Check sheet for the modelled part. Datum: model origin and axes. Units: mm. Coordinates: 2 decimals unless noted, no trailing zeros. Write each loop counter-clockwise with the first axis right and the second up, starting at its lowest first coordinate (ties: lowest second). Pieces come first, ordered by that corner, then holes. Notation, with made-up numbers: M -3.75,11 L 5.25,11 A13 cw 5.25,19 Z; hole C 86.25,-0.75 d1. An arc over 180 degrees is marked long. Answer as CSV lines item,"result". Start each with the question number.
Q1. Sectioned sample at B-B, the plane z = 58.5. Record the cut outline in (x, y), then the cut area to 3 significant figures.
Q2. Sectioned sample at A-A, the plane x = -0.5. Record the cut outline in (y, z), then the cut area to 3 significant figures.
Q3. Sectioned sample at D-D, the plane z = -27.5. Record the cut outline in (x, y), then the cut area to 3 significant figures.
Q4. Thickness scan on line 1 along Z through (x, y) = (-1.5, 0.8); line 2 along X through (y, z) = (1.75, -75) (3 decimals); line 3 along X through (y, z) = (1.85, 75). Record the ranges inside material, lowest first. Write a range as from..to.
Q5. Depth check by flat-ended pin: pin 1 Ø1.6 at (y, z) = (1, -76.5) entering from -X; pin 2 Ø1.6 at (y, z) = (2, -31) entering from +X. Enter the tip coordinate at first touch or a pass-through.
Q6. Sectioned sample at C-C, the plane x = 14.5. Record the cut outline in (y, z), then the cut area to 4 significant figures.
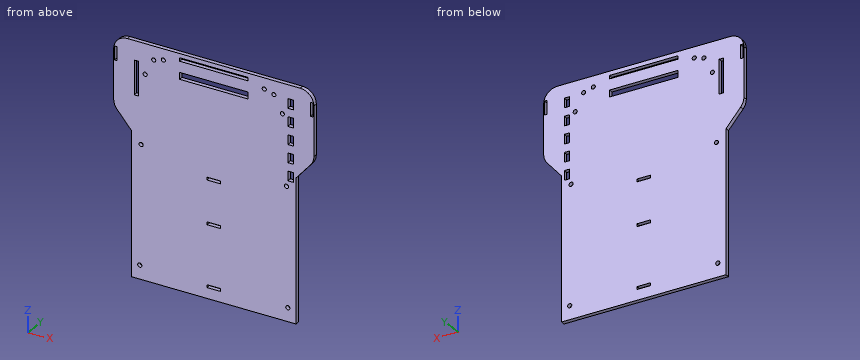
from build123d import *

# Parameters (mm, degrees)
BOSS_EXTRUDE1_DEPTH = 3
SKETCH2_R           = 1.525
CUT_EXTRUDE1_DEPTH  = 113.084789334
SKETCH3_W           = 10
SKETCH3_H           = 2.05
CUT_EXTRUDE2_DEPTH  = 113.084789334
SKETCH4_R           = 1.5
CUT_EXTRUDE3_DEPTH  = 3
SKETCH5_R           = 1.5
SKETCH5_W           = 50
SKETCH5_H           = 5
CUT_EXTRUDE4_DEPTH  = 3
SKETCH6_W           = 4
SKETCH6_H           = 7
CUT_EXTRUDE5_DEPTH  = 10
SKETCH7_W           = 50
SKETCH7_H           = 2.5
SKETCH7_W_2         = 3.05
SKETCH7_H_2         = 25
CUT_EXTRUDE6_DEPTH  = 10
FILLET3_R           = 10
SKETCH8_W           = 2
SKETCH8_H           = 10
CUT_EXTRUDE7_DEPTH  = 10


with BuildPart() as part:
    # Sketch1 → Boss-Extrude1 (new body)
    with BuildSketch(Plane(origin=(0, 0, 0), x_dir=(1, 0, 0), z_dir=(0, 1, 0))):
        Polygon((-73, -35), (-60, -19.801315846), (-60, 85), (60, 85), (60, -19.801315846), (73, -35), (73, -85), (60, -85), (-60, -85), (-73, -85), align=None)
    extrude(amount=BOSS_EXTRUDE1_DEPTH)

    # Sketch2 → Cut-Extrude1 (cut, through all)
    with BuildSketch(Plane(origin=(0, 3, 0), x_dir=(1, 0, 0), z_dir=(0, 1, 0))):
        with Locations(Location((-53, -11.81, 0), (0, 0, 270))):
            Circle(SKETCH2_R)
        with Locations(Location((-54, 75, 0), (0, 0, 270))):
            Circle(SKETCH2_R)
        with Locations(Location((53, -11.81, 0), (0, 0, 90))):
            Circle(SKETCH2_R)
        with Locations(Location((54, 75, 0), (0, 0, 90))):
            Circle(SKETCH2_R)
    extrude(amount=-CUT_EXTRUDE1_DEPTH, mode=Mode.SUBTRACT)

    # Sketch3 → Cut-Extrude2 (cut, through all)
    with BuildSketch(Plane(origin=(0, 3, 0), x_dir=(1, 0, 0), z_dir=(0, 1, 0))):
        with Locations((0, 31.115)):
            Rectangle(SKETCH3_W, SKETCH3_H)
        with Locations((0, -0.985)):
            Rectangle(SKETCH3_W, SKETCH3_H)
        with Locations((0, 76.215)):
            Rectangle(SKETCH3_W, SKETCH3_H)
    extrude(amount=-CUT_EXTRUDE2_DEPTH, mode=Mode.SUBTRACT)

    # Sketch4 → Cut-Extrude3 (cut)
    with BuildSketch(Plane(origin=(0, 3, 0), x_dir=(1, 0, 0), z_dir=(0, 1, 0))):
        with Locations(Location((-50, -63, 0), (0, 0, 270))):
            Circle(SKETCH4_R)
        with Locations(Location((-43.815341562, -75, 0), (0, 0, 270))):
            Circle(SKETCH4_R)
        with Locations(Location((43.815341562, -75, 0), (0, 0, 90))):
            Circle(SKETCH4_R)
        with Locations(Location((50, -63, 0), (0, 0, 90))):
            Circle(SKETCH4_R)
    extrude(amount=-CUT_EXTRUDE3_DEPTH, mode=Mode.SUBTRACT)

    # Sketch5 → Cut-Extrude4 (cut)
    with BuildSketch(Plane(origin=(0, 3, 0), x_dir=(1, 0, 0), z_dir=(0, 1, 0))):
        with Locations(Location((-36.8, -77, 0), (0, 0, 270))):
            Circle(SKETCH5_R)
        with Locations(Location((36.8, -77, 0), (0, 0, 90))):
            Circle(SKETCH5_R)
        with Locations((0, -69)):
            Rectangle(SKETCH5_W, SKETCH5_H)
    extrude(amount=-CUT_EXTRUDE4_DEPTH, mode=Mode.SUBTRACT)

    # Sketch6 → Cut-Extrude5 (cut)
    with BuildSketch(Plane(origin=(0, 3, 0), x_dir=(1, 0, 0), z_dir=(0, 1, 0))):
        with Locations((56, -32.549614417)):
            Rectangle(SKETCH6_W, SKETCH6_H)
        with Locations((56, -19.549614417)):
            Rectangle(SKETCH6_W, SKETCH6_H)
        with Locations((56, -45.549614417)):
            Rectangle(SKETCH6_W, SKETCH6_H)
        with Locations((56, -58.549614417)):
            Rectangle(SKETCH6_W, SKETCH6_H)
        with Locations((56, -71.549614417)):
            Rectangle(SKETCH6_W, SKETCH6_H)
    extrude(amount=-CUT_EXTRUDE5_DEPTH, mode=Mode.SUBTRACT)

    # Sketch7 → Cut-Extrude6 (cut)
    with BuildSketch(Plane(origin=(0, 3, 0), x_dir=(1, 0, 0), z_dir=(0, 1, 0))):
        with Locations((0, -80.75)):
            Rectangle(SKETCH7_W, SKETCH7_H)
        with Locations((-56.475, -58.5)):
            Rectangle(SKETCH7_W_2, SKETCH7_H_2)
    extrude(amount=-CUT_EXTRUDE6_DEPTH, mode=Mode.SUBTRACT)

    # Fillet3
    fillet3_edges = [part.edges().sort_by_distance(p)[0] for p in [
        (73, 1.5, 35),
        (73, 1.5, 85),
        (-73, 1.5, 85),
        (-73, 1.5, 35),
    ]]
    fillet(fillet3_edges, radius=FILLET3_R)

    # Sketch8 → Cut-Extrude7 (cut)
    with BuildSketch(Plane(origin=(0, 3, 0), x_dir=(1, 0, 0), z_dir=(0, 1, 0))):
        with Locations((71.5, -72)):
            Rectangle(SKETCH8_W, SKETCH8_H)
        with Locations((-71.5, -72)):
            Rectangle(SKETCH8_W, SKETCH8_H)
    extrude(amount=-CUT_EXTRUDE7_DEPTH, mode=Mode.SUBTRACT)


solid = part.part
Output:
1,outline,"M -73,0 L -58,0 L -58,3 L -73,3 Z; M -54.95,0 L 54,0 L 54,3 L -54.95,3 Z; M 58,0 L 73,0 L 73,3 L 58,3 Z"
1,area,"417 mm^2"
2,outline,"M 0,-85 L 3,-85 L 3,-77.24 L 0,-77.24 Z; M 0,-75.19 L 3,-75.19 L 3,-32.14 L 0,-32.14 Z; M 0,-30.09 L 3,-30.09 L 3,-0.04 L 0,-0.04 Z; M 0,2.01 L 3,2.01 L 3,66.5 L 0,66.5 Z; M 0,71.5 L 3,71.5 L 3,79.5 L 0,79.5 Z; M 0,82 L 3,82 L 3,85 L 0,85 Z"
2,area,"469 mm^2"
3,outline,"M -60,0 L 60,0 L 60,3 L -60,3 Z"
3,area,"360 mm^2"
4,line 1,"z = -85..-77.24, -75.19..-32.14, -30.09..-0.04, 2.01..66.5, 71.5..79.5, 82..85"
4,line 2,"x = -60..-55.525, -52.475..52.475, 55.525..60"
4,line 3,"x = -73..-72.5, -70.5..-45.32, -42.32..42.32, 45.32..54, 58..70.5, 72.5..73"
5,pin 1,"stops at x = -60"
5,pin 2,"stops at x = 60"
6,outline,"M 0,-85 L 3,-85 L 3,66.5 L 0,66.5 Z; M 0,71.5 L 3,71.5 L 3,79.5 L 0,79.5 Z; M 0,82 L 3,82 L 3,85 L 0,85 Z"
6,area,"487.5 mm^2"
